Geometry check sheet. Reference: the model listing, model coordinates, mm. Round coordinates to 2 decimals unless told otherwise and drop trailing zeros. Order: outer loops, then holes, each group sorted by start corner. A loop starts at its lowest first (then second) coordinate and runs counter-clockwise, first axis right, second up. Notation, with made-up numbers: (53.25, -15) - (69.25, -15) arc R23 ccw to (69.25, 23) - close; hole circle Ø4 at (26.5, 74). An arc over 180 degrees is marked (long way). One line per question, with ' | ' between items. Start each with the question number.
Q1. Sectioned sample at D-D, the plane x = 3.1. Enter the section's corners in (y, z).
Q2. Material ranges on line 1 along Y through (x, z) = (15.25, 0.8); line 2 along Y through (x, z) = (3.1, 0.85); line 3 along X through (y, z) = (31.5, 1.45), recorded low to high.
Q3. Sectioned sample at B-B, the plane x = 15.25. Enter the section's corners in (y, z), then the cut area to 3 significant figures.
Q4. Gauge pin test, flat ends, axial feed: P1, Ø0.6, axis at x = -14.5, z = 0.5, coming from the +Y side; P2, Ø1, axis at y = 25, z = 0.5, coming from the -X side. Record the tip position at first contact, or that the pin passes through.
Q5. Sectioned sample at A-A, the plane y = 31.6. Enter the section's corners in (x, z), then the cut area to 3 significant figures.
Q6. Sectioned sample at C-C, the plane z = 0.35. Enter the section's corners in (x, y), then the cut area to 3 significant figures.
```python
from build123d import *

# Parameters (mm, degrees)
F0_R     = 1.5
F0_W     = 14.8
F0_H     = 17.9
F1_DEPTH = 2


with BuildPart() as f1:
    # F0 (on Top) → F1 (new body)
    with BuildSketch(Plane.XY):
        Polygon((-7.4, 18), (-18, 18), (-18, -18), (18, -18), (18, 18), (7.4, 18), align=None)
        with Locations((-15.25, -15.25)):
            Circle(F0_R, mode=Mode.SUBTRACT)
        with Locations((15.25, -15.25)):
            Circle(F0_R, mode=Mode.SUBTRACT)
        with Locations((-15.25, 15.25)):
            Circle(F0_R, mode=Mode.SUBTRACT)
        with Locations((15.25, 15.25)):
            Circle(F0_R, mode=Mode.SUBTRACT)
        with Locations((0, 26.95)):
            Rectangle(F0_W, F0_H)
        with Locations((-3.08587, 31.6)):
            Circle(F0_R, mode=Mode.SUBTRACT)
        with Locations((3.1, 31.6)):
            Circle(F0_R, mode=Mode.SUBTRACT)
    extrude(amount=F1_DEPTH)


solid = f1.part
```
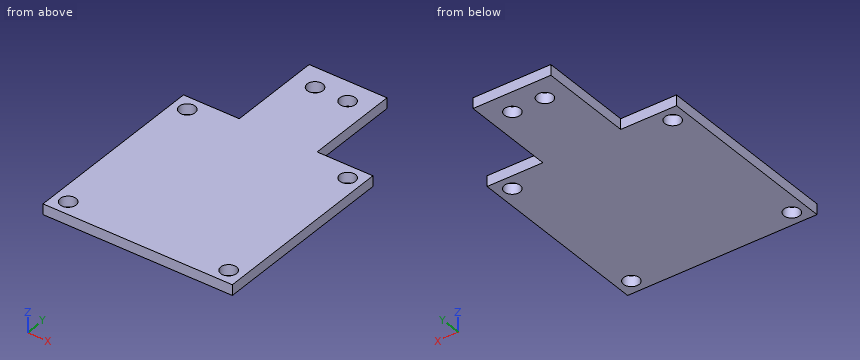
Determined:
1) outline: (-18, 0) - (30.1, 0) - (30.1, 2) - (-18, 2) - close; (33.1, 0) - (35.9, 0) - (35.9, 2) - (33.1, 2) - close
2) line 1: y = -18 to -16.75, -13.75 to 13.75, 16.75 to 18 | line 2: y = -18 to 30.1, 33.1 to 35.9 | line 3: x = -7.4 to -4.58, -1.59 to 1.6, 4.6 to 7.4
3) outline: (-18, 0) - (-16.75, 0) - (-16.75, 2) - (-18, 2) - close; (-13.75, 0) - (13.75, 0) - (13.75, 2) - (-13.75, 2) - close; (16.75, 0) - (18, 0) - (18, 2) - (16.75, 2) - close | area: 60.0 mm2
4) P1: stops at y = 18 | P2: stops at x = -7.4
5) outline: (-7.4, 0) - (-4.59, 0) - (-4.59, 2) - (-7.4, 2) - close; (-1.59, 0) - (1.6, 0) - (1.6, 2) - (-1.59, 2) - close; (4.6, 0) - (7.4, 0) - (7.4, 2) - (4.6, 2) - close | area: 17.6 mm2
6) outline: (-18, -18) - (18, -18) - (18, 18) - (7.4, 18) - (7.4, 35.9) - (-7.4, 35.9) - (-7.4, 18) - (-18, 18) - close; hole circle Ø3 at (-15.25, -15.25); hole circle Ø3 at (-15.25, 15.25); hole circle Ø3 at (-3.09, 31.6); hole circle Ø3 at (3.1, 31.6); hole circle Ø3 at (15.25, -15.25); hole circle Ø3 at (15.25, 15.25) | area: 1,520 mm2
